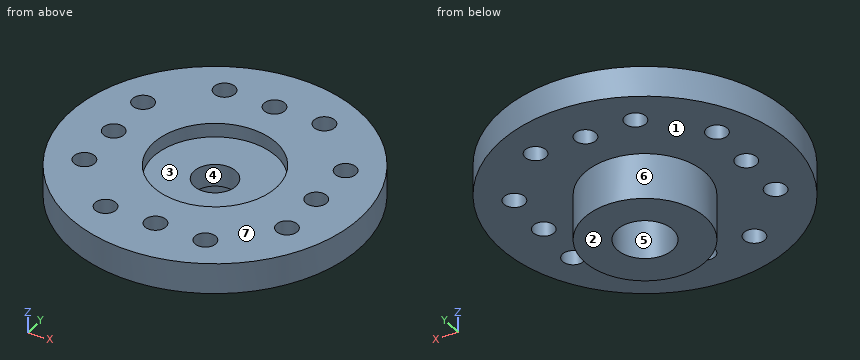
```python
from build123d import *

# Parameters (mm, degrees)
SKETCH_1_R          = 10.4
EXTRUDE_1_DEPTH     = 2.2
SKETCH_2_R          = 4.35
EXTRUDE_2_DEPTH     = 3.3
CUT_EXTRUDE_START   = 3.3
SKETCH_3_R          = 1.5
CUT_EXTRUDE_1_DEPTH = 19.373486657
SKETCH_4_R          = 4.4
CUT_EXTRUDE_2_DEPTH = 1
SKETCH_5_R          = 0.75
CUT_EXTRUDE_3_DEPTH = 16.702547564
SKETCH_6_R          = 2
CUT_EXTRUDE_4_DEPTH = 2.9


with BuildPart() as part:
    # 草图1 → 凸台-拉伸1 (new body)
    with BuildSketch(Plane.XY):
        Circle(SKETCH_1_R)
    extrude(amount=EXTRUDE_1_DEPTH)

    # 草图2 → 凸台-拉伸2 (add)
    with BuildSketch(Plane(origin=(0, 0, 0), x_dir=(-1, 0, 0), z_dir=(0, 0, -1))):
        Circle(SKETCH_2_R)
    extrude(amount=EXTRUDE_2_DEPTH)

    # 草图3 → 切除-拉伸1 (cut, through all)
    with BuildSketch(Plane(origin=(0, 0, 0), x_dir=(-1, 0, 0), z_dir=(0, 0, -1)).offset(CUT_EXTRUDE_START)):
        Circle(SKETCH_3_R)
    extrude(amount=-CUT_EXTRUDE_1_DEPTH, mode=Mode.SUBTRACT)

    # 草图4 → 切除-拉伸2 (cut)
    with BuildSketch(Plane.XY.offset(2.2)):
        Circle(SKETCH_4_R)
    extrude(amount=-CUT_EXTRUDE_2_DEPTH, mode=Mode.SUBTRACT)

    # 草图5 → 切除-拉伸3 (cut, through all)
    with BuildSketch(Plane.XY.offset(2.2)):
        with Locations((0, 7.1)):
            Circle(SKETCH_5_R)
        with Locations((3.5, 7.1)):
            Circle(SKETCH_5_R)
        with Locations((-3.5, 7.1)):
            Circle(SKETCH_5_R)
        with Locations((7.1, 3.5)):
            Circle(SKETCH_5_R)
        with Locations((7.1, 0)):
            Circle(SKETCH_5_R)
        with Locations((7.1, -3.5)):
            Circle(SKETCH_5_R)
        with Locations((3.5, -7.1)):
            Circle(SKETCH_5_R)
        with Locations((0, -7.1)):
            Circle(SKETCH_5_R)
        with Locations((-3.5, -7.1)):
            Circle(SKETCH_5_R)
        with Locations((-7.1, -3.5)):
            Circle(SKETCH_5_R)
        with Locations((-7.1, 0)):
            Circle(SKETCH_5_R)
        with Locations((-7.1, 3.5)):
            Circle(SKETCH_5_R)
    extrude(amount=-CUT_EXTRUDE_3_DEPTH, mode=Mode.SUBTRACT)

    # 草图6 → 切除-拉伸4 (cut)
    with BuildSketch(Plane(origin=(0, 0, -3.3), x_dir=(-1, 0, 0), z_dir=(0, 0, -1))):
        Circle(SKETCH_6_R)
    extrude(amount=-CUT_EXTRUDE_4_DEPTH, mode=Mode.SUBTRACT)


solid = part.part
```
Part model, mm, in its own coordinate system. Face numbers are marked on the shaded views. A direction names the side the tool comes from. Give positions to 0.01 mm unless a question says otherwise; leave off trailing zeros. Order: outer loops, then holes, each group sorted by start corner. A loop starts at its lowest first (then second) coordinate and runs counter-clockwise, first axis right, second up. Notation, with made-up numbers: M -27.75,-4 L -7.75,-4 A22 ccw -7.75,17 Z; hole C -4,55.25 d11. An arc over 180 degrees is marked long. Use a Markdown table: item, result. Add a question column.
(1) Saw through at B-B, the plane y = -4. Give the cut face in (x, z), and give its area (3 significant figures).
(2) Probe line 1 along Y through (x, z) = (0, 1.55); line 2 along Y through (x, z) = (-3.75, 0.2); line 3 along Y through (x, z) = (3.5, 1.55). List the from-to ranges inside material, lowest first. Write a range as [from, to].
(3) Mould opens along X. For the marked faces 4, 5, 6 and 7 say: +X half, -X half, draft (parallel to the pull), parting line (faces both ways), or undercut.
(4) 3-axis set-ups, long thin cutter, end or side, ignore diameter. For the marked faces 1, 2 and 3: which of +Z, -Z, +X, -X, +Y, -Y reach the whole face in a straight line?
(5) Saw through at D-D, the plane x = 6.75. Give the cut face in (y, z), and give its area (3 significant figures).
(6) Saw through at A-A, the plane x = 3.5. Give the cut face in (y, z).
(7) Saw through at C-C, the plane y = 0.5. Give the cut face in (x, z).
(8) Drop flat-ended pins along their axis: P1, Ø1.4, axis at x = 3.5, y = -7.1, coming from the -Z side; P2, Ø2, axis at x = -3.5, y = -7.1, coming from the -Z side. Give the stop position or say it passes through.
Answer key:
| question | item | result |
|---|---|---|
| 1 | outline | M -9.6,0 L -7.66,0 L -7.66,2.2 L -9.6,2.2 Z; M -6.54,0 L -1.71,0 L -1.71,-3.3 L 1.71,-3.3 L 1.71,0 L 6.54,0 L 6.54,2.2 L 1.83,2.2 L 1.83,1.2 L -1.83,1.2 L -1.83,2.2 L -6.54,2.2 Z; M 7.66,0 L 9.6,0 L 9.6,2.2 L 7.66,2.2 Z |
| 1 | area | 44.9 mm^2 |
| 2 | line 1 | [-10.4, -7.85], [-6.35, -4.4], [4.4, 6.35], [7.85, 10.4] |
| 2 | line 2 | [-9.7, -7.81], [-6.39, 6.39], [7.81, 9.7] |
| 2 | line 3 | [-9.79, -7.85], [-6.35, -2.67], [2.67, 6.35], [7.85, 9.79] |
| 3 | face 4 | undercut |
| 3 | face 5 | undercut |
| 3 | face 6 | parting line |
| 3 | face 7 | draft |
| 4 | face 1 | -Z |
| 4 | face 2 | -Z, +X, -X, +Y, -Y |
| 4 | face 3 | +Z |
| 5 | outline | M -7.91,0 L -4.16,0 L -4.16,2.2 L -7.91,2.2 Z; M -2.84,0 L -0.66,0 L -0.66,2.2 L -2.84,2.2 Z; M 0.66,0 L 2.84,0 L 2.84,2.2 L 0.66,2.2 Z; M 4.16,0 L 7.91,0 L 7.91,2.2 L 4.16,2.2 Z |
| 5 | area | 26.1 mm^2 |
| 6 | outline | M -9.79,0 L -7.85,0 L -7.85,2.2 L -9.79,2.2 Z; M -6.35,0 L -2.58,0 L -2.58,-3.3 L 2.58,-3.3 L 2.58,0 L 6.35,0 L 6.35,2.2 L 2.67,2.2 L 2.67,1.2 L -2.67,1.2 L -2.67,2.2 L -6.35,2.2 Z; M 7.85,0 L 9.79,0 L 9.79,2.2 L 7.85,2.2 Z |
| 7 | outline | M -10.39,0 L -7.66,0 L -7.66,2.2 L -10.39,2.2 Z; M -6.54,0 L -4.32,0 L -4.32,-3.3 L -1.94,-3.3 L -1.94,-0.4 L -1.41,-0.4 L -1.41,1.2 L -4.37,1.2 L -4.37,2.2 L -6.54,2.2 Z; M 1.41,-0.4 L 1.94,-0.4 L 1.94,-3.3 L 4.32,-3.3 L 4.32,0 L 6.54,0 L 6.54,2.2 L 4.37,2.2 L 4.37,1.2 L 1.41,1.2 Z; M 7.66,0 L 10.39,0 L 10.39,2.2 L 7.66,2.2 Z |
| 8 | P1 | through |
| 8 | P2 | z = 0 |
